Geometry check sheet. Reference: the model listing, model coordinates, mm. A direction names the side the tool comes from. Give positions to 0.01 mm unless a question says otherwise; leave off trailing zeros. Loops run counter-clockwise (first coordinate to the right, second up) from the corner with the lowest first, then second, coordinate; pieces in that order, holes last. Notation, with made-up numbers: (-14.75, -34.5) - (-2.75, -34.5) arc R17 ccw to (-2.75, -29.5) - close; hole circle Ø2 at (-32.5, -32). An arc over 180 degrees is marked (long way). Use a Markdown table: item, result. Add a question column.
1. Cross-section at D-D on x = 0. Enter the section's corners in (y, z), and give its area (3 significant figures).
2. Set-up check for faces 1 (the cylindrical face through (0.443, -19.66, -25.396)), 2 (the flat face through (-31, -20, -6.35)), 3 (the cylindrical face through (19.73, -20.22, -0.66)): record each of +Z, -Z, +X, -X, +Y, -Y from which the full face is reachable in a straight line by a thin tool's end or side.
3. Cross-section at A-A on z = -3.25. Enter the section's corners in (x, y) (1 decimal), and give its area (3 significant figures).
4. Depth check by flat-ended pin: P1, Ø10, axis at y = -17, z = -20.5, coming from the +X side; P2, Ø8, axis at x = -30.16, y = -32.64, coming from the +Z side; P3, Ø4, axis at y = -25, z = -20, coming from the +X side; P4, Ø10, axis at y = -23, z = -13.5, coming from the +X side. Enter the tip coordinate at first touch or a pass-through.
5. Draft check along X on faces 4 (the cylindrical face through (-28.35, -30.98, -3.13)), 5 (the flat face through (-0.2, 0, -19.3)), 6 (the cylindrical face through (25.023, -20.218, -6.815)), 7 (the cylindrical face through (-34.201, -0.764, -3.131)). Enter one of: pulls with the +X half, pulls with the -X half, needs draft (parallel to the pull), parting line crosses it, or undercut.
6. Material ranges on L1, parallel to X at y = -5.5, z = -4 (3 decimals); L2, parallel to X at y = -12, z = -15.25; L3, parallel to Z at x = -27, y = -20, recorded low to high.
7. Cross-section at C-C on y = -23.5. Enter the section's corners in (x, z) (3 decimals), and give its area (3 significant figures).
8. Cross-section at B-B on z = -9.5. Enter the section's corners in (x, y), and give its area (3 significant figures).
from build123d import *

# Parameters (mm, degrees)
BOSS_EXTRUDE2_DEPTH          = 39.878
FILLET1_R                    = 2.54
F_10_0_1935_DIAMETER_HOLE1_D = 4.9149


with BuildPart() as part:
    # Sketch5 → Boss-Extrude2 (new body)
    with BuildSketch(Plane(origin=(0, 0, 0), x_dir=(1, 0, 0), z_dir=(0, 1, 0))):
        with BuildLine():
            Line((-34.925, 0), (-19.05, 0))
            ThreePointArc((-19.05, 0), (0, 19.05), (19.05, 0))
            Line((19.05, 0), (34.925, 0))
            Line((34.925, 0), (34.925, 6.35))
            Line((34.925, 6.35), (24.593444248, 6.35))
            ThreePointArc((24.593444248, 6.35), (0, 25.4), (-24.593444248, 6.35))
            Line((-24.593444248, 6.35), (-34.925, 6.35))
            Line((-34.925, 6.35), (-34.925, 0))
        make_face()
    extrude(amount=-BOSS_EXTRUDE2_DEPTH)

    # Fillet1
    fillet1_edges = [part.edges().sort_by_distance(p)[0] for p in [
        (-34.925, 0, -3.175),
        (-24.593444248, -19.939, -6.35),
        (24.593444248, -19.939, -6.35),
        (19.05, -19.939, 0),
        (-19.05, -19.939, 0),
        (34.925, -39.878, -3.175),
        (-34.925, -39.878, -3.175),
        (34.925, 0, -3.175),
    ]]
    fillet(fillet1_edges, radius=FILLET1_R)

    # #10 (0.1935) Diameter Hole1 (through all)
    with Locations(Plane(origin=(0, 0, -6.35), x_dir=(-1, 0, 0), z_dir=(0, 0, -1))):
        with Locations((-30.1625, -7.239), (-30.1625, -32.639)):
            f_10_0_1935_diameter_hole1 = Hole(F_10_0_1935_DIAMETER_HOLE1_D / 2)

    # Mirror1: #10 (0.1935) Diameter Hole1 across plane
    add(f_10_0_1935_diameter_hole1.mirror(Plane(origin=(0, 0, 0), x_dir=(0, 0, 1), z_dir=(1, 0, 0))), mode=Mode.SUBTRACT)


solid = part.part
Values found:
| question | item | result |
|---|---|---|
| 1 | outline | (-39.88, -25.4) - (0, -25.4) - (0, -19.05) - (-39.88, -19.05) - close |
| 1 | area | 253 mm2 |
| 2 | face 1 | -Z, +Y, -Y |
| 2 | face 2 | -Z, -X, +Y, -Y |
| 2 | face 3 | +Z, +Y, -Y |
| 3 | outline | (-34.9, -37.3) arc R2.5 ccw to (-32.4, -39.9) - (-18.8, -39.9) - (-18.8, 0) - (-32.4, 0) arc R2.5 ccw to (-34.9, -2.5) - close; (18.8, -39.9) - (32.4, -39.9) arc R2.5 ccw to (34.9, -37.3) - (34.9, -2.5) arc R2.5 ccw to (32.4, 0) - (18.8, 0) - close; hole circle Ø4.9 at (-30.2, -32.6); hole circle Ø4.9 at (-30.2, -7.2); hole circle Ø4.9 at (30.2, -32.6); hole circle Ø4.9 at (30.2, -7.2) |
| 3 | area | 1,210 mm2 |
| 4 | P1 | stops at x = 20.12 |
| 4 | P2 | stops at z = 0 |
| 4 | P3 | stops at x = 17.92 |
| 4 | P4 | stops at x = 23.94 |
| 5 | face 4 | undercut |
| 5 | face 5 | needs draft |
| 5 | face 6 | pulls with the +X half |
| 5 | face 7 | pulls with the -X half |
| 6 | L1 | x = -34.925 to -31.899, -28.426 to -18.625, 18.625 to 28.426, 31.899 to 34.925 |
| 6 | L2 | x = -20.31 to -11.42, 11.42 to 20.31 |
| 6 | L3 | z = -6.35 to 0 |
| 7 | outline | (-34.925, -6.35) - (-26.488, -6.35) arc R2.54 cw to (-24.08, -8.082) arc R25.4 ccw to (24.08, -8.082) arc R2.54 cw to (26.488, -6.35) - (34.925, -6.35) - (34.925, 0) - (21.44, 0) arc R2.54 ccw to (18.918, -2.241) arc R19.05 cw to (-18.918, -2.241) arc R2.54 ccw to (-21.44, 0) - (-34.925, 0) - close |
| 7 | area | 567 mm2 |
| 8 | outline | (-23.56, -39.88) - (-16.51, -39.88) - (-16.51, 0) - (-23.56, 0) - close; (16.51, -39.88) - (23.56, -39.88) - (23.56, 0) - (16.51, 0) - close |
| 8 | area | 562 mm2 |
